Part model, mm, in its own coordinate system. A direction names the side the tool comes from. Round coordinates to 2 decimals unless told otherwise and drop trailing zeros. Loops run counter-clockwise (first coordinate to the right, second up) from the corner with the lowest first, then second, coordinate; pieces in that order, holes last.
from build123d import *

# Parameters (mm, degrees)
F0_W     = 56.9855384529
F0_H     = 6.0439207591
F1_DEPTH = 38.1
F3_DEPTH = 12.7
F4_R     = 5.6337267147
F5_DEPTH = 25.4
F6_R     = 2.5763739366
F6_R_2   = 2.4951731212
F6_R_3   = 2.3565031445
F7_DEPTH = 25.4


with BuildPart() as f1:
    # F0 (on Front) → F1 (new body)
    with BuildSketch(Plane.XZ):
        with Locations((28.4927692264, 3.0219603796)):
            Rectangle(F0_W, F0_H)
    extrude(amount=F1_DEPTH)

    # F2 (on Front) → F3 (join)
    with BuildSketch(Plane.XZ):
        Polygon((0, 44.45), (0, 0), (38.1, 0), (38.1, 12.7), (25.4, 12.7), (25.4, 44.45), align=None)
    extrude(amount=F3_DEPTH)

    # F4 (on face) → F5 (cut)
    with BuildSketch(Plane.XZ.offset(12.7)):
        with BuildLine():
            ThreePointArc((0, 31.75), (12.7, 43.757902847), (25.4, 31.75))
            Line((25.4, 31.75), (25.4, 44.45))
            Line((25.4, 44.45), (0, 44.45))
            Line((0, 44.45), (0, 31.75))
        make_face()
        with Locations((12.7, 31.75)):
            Circle(F4_R)
        with BuildLine():
            Line((38.1, 12.7), (25.4, 12.7))
            ThreePointArc((25.4, 12.7), (30.9307359014, 7.8087797629), (38.1, 6.0439207591))
            Line((38.1, 6.0439207591), (38.1, 12.7))
        make_face()
    extrude(amount=-F5_DEPTH, mode=Mode.SUBTRACT)

    # F6 (on face) → F7 (cut)
    with BuildSketch(Plane.XY.offset(6.0439207591)):
        with BuildLine():
            ThreePointArc((56.9855384529, -33.4053455879), (55.411700833, -36.5261623801), (52.2908840407, -38.1))
            Line((52.2908840407, -38.1), (56.9855384529, -38.1))
            Line((56.9855384529, -38.1), (56.9855384529, -33.4053455879))
        make_face()
        with BuildLine():
            ThreePointArc((5.0487379712, -38.1), (1.6431313477, -36.4568686523), (0, -33.0512620288))
            Line((0, -33.0512620288), (0, -38.1))
            Line((0, -38.1), (5.0487379712, -38.1))
        make_face()
        with Locations((51.4632112468, -10.8606727939)):
            Circle(F6_R)
        with Locations((51.4632112468, -32.5776727939)):
            Circle(F6_R_2)
        with Locations((5.6993689856, -32.4006310144)):
            Circle(F6_R_3)
    extrude(amount=-F7_DEPTH, mode=Mode.SUBTRACT)


solid = f1.part
1) Mould opens along Z. For faces 4 (the face through (15, -12.7, 21)), 5 (the face through (30.838, -6.439, 7.858)), 6 (the face through (28, -19, 0)), 7 (the face through (18.074, -6.439, 33.442)) say: released by +Z, released by -Z, zero draft, split by the parting line, or undercut.
Values:
face 4: zero draft
face 5: released by +Z
face 6: released by -Z
face 7: undercut
2) Slice it at C-C, the plane z = 30. Give the cut face in (x, y).
Values:
outline: (0, -12.7) - (7.34, -12.7) - (7.34, 0) - (0, 0) - close; (18.06, -12.7) - (25.4, -12.7) - (25.4, 0) - (18.06, 0) - close
3) Wall check: line 1 along Z through (x, y) = (12, -31.5); line 2 along Y through (x, z) = (9.5, 7.5); line 3 along Z through (x, y) = (32, -3). Give the ranges that are in metal, low to high.
Values:
line 1: z = 0 to 6.04
line 2: y = -12.7 to 0
line 3: z = 0 to 7.3
4) Drop flat-ended pins along their axis: pin 1 Ø14 at (y, z) = (-4, 26) entering from +X; pin 2 Ø10 at (x, z) = (8, 18.5) entering from -Y. Give the stop position or say it passes through.
Values:
pin 1: stops at x = 25.4
pin 2: stops at y = -12.7
5) Slice it at B-B, the plane y = -31.5. Give the cut face in (x, z), then the cut area to 3 significant figures.
Values:
outline: (0, 0) - (3.52, 0) - (3.52, 6.04) - (0, 6.04) - close; (7.88, 0) - (49.21, 0) - (49.21, 6.04) - (7.88, 6.04) - close; (53.71, 0) - (56.99, 0) - (56.99, 6.04) - (53.71, 6.04) - close
area: 291 mm2
6) Tool access for faces 1 (the face through (25.4, -6, 22)), 2 (the face through (0, -9, 13)), 3 (the face through (28, -23, 6.044)): list every direction of +Z, -Z, +X, -X, +Y, -Y with a clear straight run to the whole face (end or side of a thin tool).
Values:
face 1: +Z, +X, +Y, -Y
face 2: +Z, -Z, -X, +Y, -Y
face 3: +Z, +X, -Y
7) Slice it at D-D, the plane x = 6. Give the cut face in (y, z), then the cut area to 3 significant figures.
Values:
outline: (-38.1, 0) - (-34.74, 0) - (-34.74, 6.04) - (-38.1, 6.04) - close; (-30.06, 0) - (0, 0) - (0, 41.85) - (-12.7, 41.85) - (-12.7, 6.04) - (-30.06, 6.04) - close
area: 657 mm2
8) Slice it at A-A, the plane x = 12.7. Give the cut face in (y, z), then the cut area to 3 significant figures.
Values:
outline: (-38.1, 0) - (0, 0) - (0, 26.12) - (-12.7, 26.12) - (-12.7, 6.04) - (-38.1, 6.04) - close; (-12.7, 37.38) - (0, 37.38) - (0, 43.76) - (-12.7, 43.76) - close
area: 566 mm2
